from build123d import *

# Parameters (mm, degrees)
SKETCH2_R           = 12.7
BOSS_EXTRUDE1_DEPTH = 25.4
CHAMFER1_SIZE       = 1.905


with BuildPart() as part:
    # Sketch2 → Boss-Extrude1 (new body)
    with BuildSketch(Plane(origin=(0, 0, 0), x_dir=(1, 0, 0), z_dir=(0, 1, 0))):
        with BuildLine():
            Line((63.5, 25.4), (98.373776994, 25.4))
            ThreePointArc((98.373776994, 25.4), (74.143548783, 69.464337424), (31.75, 96.511644375))
            Line((31.75, 96.511644375), (31.75, 63.5))
            ThreePointArc((31.75, 63.5), (0, 31.75), (-31.75, 63.5))
            Line((-31.75, 63.5), (-31.75, 96.511644375))
            ThreePointArc((-31.75, 96.511644375), (-78.413523495, 64.605567354), (-100.803124952, 12.7))
            Line((-100.803124952, 12.7), (-63.5, 12.7))
            ThreePointArc((-63.5, 12.7), (-50.8, 0), (-63.5, -12.7))
            Line((-63.5, -12.7), (-100.803124952, -12.7))
            ThreePointArc((-100.803124952, -12.7), (-74.079092421, -69.533071743), (-19.05, -99.798083649))
            Line((-19.05, -99.798083649), (-19.05, -63.5))
            ThreePointArc((-19.05, -63.5), (0, -44.45), (19.05, -63.5))
            Line((19.05, -63.5), (19.05, -99.798083649))
            ThreePointArc((19.05, -99.798083649), (69.504349242, -74.106041835), (98.373776994, -25.4))
            Line((98.373776994, -25.4), (63.5, -25.4))
            ThreePointArc((63.5, -25.4), (38.1, 0), (63.5, 25.4))
        make_face()
        with Locations(Location((0, 0, 0), (0, 0, 270))):
            Circle(SKETCH2_R, mode=Mode.SUBTRACT)
    extrude(amount=BOSS_EXTRUDE1_DEPTH)

    # Chamfer1
    chamfer1_edges = [part.edges().sort_by_distance(p)[0] for p in [
        (74.143548783, 25.4, -69.464337424),
        (80.936888497, 0, 25.4),
        (69.504349242, 0, 74.106041835),
        (19.05, 0, 81.649041824),
        (31.75, 25.4, -80.005822188),
        (0, 0, 44.45),
        (-19.05, 0, 81.649041824),
        (-74.079092421, 0, 69.533071743),
        (-82.151562476, 0, 12.7),
        (-50.8, 0, 0),
        (-82.151562476, 0, -12.7),
        (-78.413523495, 0, -64.605567354),
        (-31.75, 0, -80.005822188),
        (0, 0, -31.75),
        (31.75, 0, -80.005822188),
        (0, 25.4, -31.75),
        (74.143548783, 0, -69.464337424),
        (80.936888497, 0, -25.4),
        (38.1, 0, 0),
        (-31.75, 25.4, -80.005822188),
        (-78.413523495, 25.4, -64.605567354),
        (-82.151562476, 25.4, -12.7),
        (-50.8, 25.4, 0),
        (0, 0, -12.7),
        (0, 25.4, -12.7),
        (-82.151562476, 25.4, 12.7),
        (-74.079092421, 25.4, 69.533071743),
        (-19.05, 25.4, 81.649041824),
        (38.1, 25.4, 0),
        (0, 25.4, 44.45),
        (19.05, 25.4, 81.649041824),
        (69.504349242, 25.4, 74.106041835),
        (80.936888497, 25.4, 25.4),
        (80.936888497, 25.4, -25.4),
    ]]
    chamfer(chamfer1_edges, length=CHAMFER1_SIZE)


solid = part.part
Could you check a few things on this model? Use its own coordinates, in mm. A direction names the side the tool comes from. Round coordinates to 2 decimals unless told otherwise and drop trailing zeros. Order: outer loops, then holes, each group sorted by start corner. A loop starts at its lowest first (then second) coordinate and runs counter-clockwise, first axis right, second up.
Q1. Please list where these lines run through material, in increasing order: probe 1 along X at (y, z) = (13, -1); probe 2 along X at (y, z) = (20, 51.5); probe 3 along Z at (x, y) = (-72, 24.25) (3 decimals).
Geometry says:
probe 1: x = -50.84 to -12.66, 12.66 to 38.12
probe 2: x = -87.58 to -14.8, 14.8 to 87.58
probe 3: z = -70.61 to -13.455, 13.455 to 70.61
Q2. Which directions (+Z, -Z, +X, -X, +Y, -Y) give clear straight access to the entire face, cutting with the end or side of a thin tool? Please do faces 5 (the face through (81, 13, -25.4)), 6 (the face through (73.452, 0.304, -67.857)), 7 (the face through (31.75, 13, -80)), 8 (the face through (19.05, 13, 81)).
Geometry says:
face 5: +X, +Y, -Y
face 6: -Z, +X, -Y
face 7: -Z, +Y, -Y
face 8: +Z, +Y, -Y
Q3. Thinking about a two-plate mould opening in Z: for faces 1 (the face through (81, 13, 25.4)), 2 (the face through (-50.684, 23.614, -0.282)), 3 (the face through (-73.5, 0.3, 67.8)), 4 (the face through (-76.67, 0.3, -64.19)), which applies, released by +Z, released by -Z, zero draft, split by the parting line, or undercut?
Geometry says:
face 1: undercut
face 2: undercut
face 3: released by +Z
face 4: released by -Z
Q4. Imagine slicing it at A-A, the plane y = 11.5. List the corners of the cut face in (x, z) for me.
Geometry says:
outline: (-100.8, -12.7) arc R101.6 ccw to (-31.75, -96.51) - (-31.75, -63.5) arc R31.75 cw to (31.75, -63.5) - (31.75, -96.51) arc R101.6 ccw to (98.37, -25.4) - (63.5, -25.4) arc R25.4 cw to (63.5, 25.4) - (98.37, 25.4) arc R101.6 ccw to (19.05, 99.8) - (19.05, 63.5) arc R19.05 cw to (-19.05, 63.5) - (-19.05, 99.8) arc R101.6 ccw to (-100.8, 12.7) - (-63.5, 12.7) arc R12.7 cw to (-63.5, -12.7) - close; hole circle Ø25.4 at (0, 0)
Q5. Imagine slicing it at B-B, the plane x = 0. List the corners of the cut face in (y, z) for me (3 decimals), then the cut area to 3 significant figures.
Geometry says:
outline: (0, -29.845) - (1.905, -31.75) - (23.495, -31.75) - (25.4, -29.845) - (25.4, -14.605) - (23.495, -12.7) - (1.905, -12.7) - (0, -14.605) - close; (0, 14.605) - (1.905, 12.7) - (23.495, 12.7) - (25.4, 14.605) - (25.4, 42.545) - (23.495, 44.45) - (1.905, 44.45) - (0, 42.545) - close
area: 1,280 mm2
Q6. I'm going to push flat-ended pins straight in: P1, Ø6, axis at x = -79.5, y = 9, coming from the +Z side; P2, Ø10, axis at x = -18.5, z = 54.5, coming from the -Y side; P3, Ø11, axis at y = 18, z = 73.5, coming from the +X side; P4, Ø5, axis at x = 35, y = 2.5, coming from the -Z side. Where does each tip first touch, or does it pass through?
Geometry says:
P1: stops at z = 66.86
P2: stops at y = 0
P3: stops at x = 75.49
P4: stops at z = -96.26
